Can you work these out from the model? Positions are in its coordinate system, mm. Give positions to 0.01 mm unless a question says otherwise; leave off trailing zeros. Loops run counter-clockwise (first coordinate to the right, second up) from the corner with the lowest first, then second, coordinate; pieces in that order, holes last. Notation, with made-up numbers: (-31, 25) - (10, 25) arc R5 ccw to (10, 31) - close; hole circle Ø3 at (82.5, 36.5). An arc over 180 degrees is marked (long way). Answer as a JSON object with one key per item and string values.
Autodesk Inventor part; units mm, degrees
ref_plane "YZ Plane" through (0, 0, 0) normal (1, 0, 0) x (0, 1, 0)
ref_plane "XZ Plane" through (0, 0, 0) normal (0, 1, 0) x (-1, 0, 0)
ref_plane "XY Plane" through (0, 0, 0) normal (0, 0, 1) x (1, 0, 0)
sketch "Sketch1" plane through (0, 0, 0) normal (0, 1, 0) x (-1, 0, 0)
  line L0 (0, 0) -> (120, 0)
  line L1 (120, 0) -> (120, -40)
  line L2 (120, -40) -> (0, -40)
  line L3 (0, -40) -> (0, 0)
  circle A0 centre (10, -20) radius 3
  circle A1 centre (110, -10) radius 3
  circle A2 centre (110, -30) radius 3
  dimension "d0" = 120
  dimension "d1" = 40
  dimension "d2" = 6
  dimension "d3" = 10
  dimension "d4" = 20
  dimension "d5" = 6
  dimension "d6" = 10
  dimension "d7" = 6
  dimension "d8" = 20
  dimension "d9" = 10
  dimension "d10" = 10
extrude "Extrusion1" add sketch "Sketch1" along normal blind 6
fillet "Fillet1" radius 5 4 edges at (0, 3, 0) (0, 3, -40) (-120, 3, 0) (-120, 3, -40)
properties part number "EboxTslotMount"
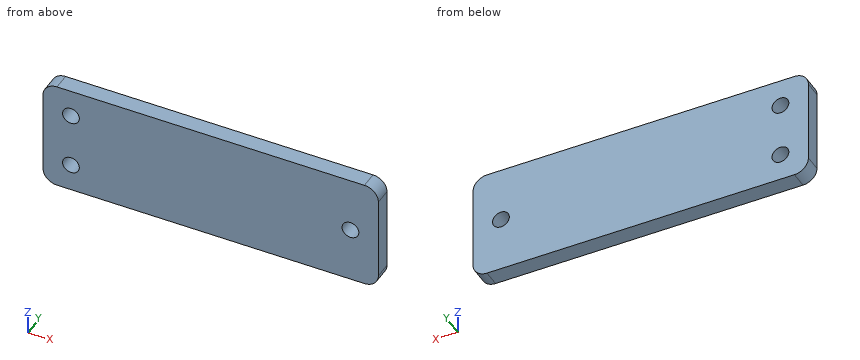
1) I need wall thicknesses on L1, parallel to Z at x = -110, y = 1.75; L2, parallel to Z at x = -10, y = 4.05; L3, parallel to X at y = 3.3, z = -21. Which ranges of each line are inside material? Lowest first, please.
Check sheet entries:
{"L1": "-40 to -33, -27 to -13, -7 to 0", "L2": "-40 to -23, -17 to 0", "L3": "-120 to -12.83, -7.17 to 0"}
2) Imagine slicing it at B-B on x = -10. Write out the boundary of the cut face in (y, z), and give its area (3 significant figures).
Check sheet entries:
{"outline": "(0, -40) - (6, -40) - (6, -23) - (0, -23) - close; (0, -17) - (6, -17) - (6, 0) - (0, 0) - close", "area": "204 mm2"}
3) Imagine slicing it at D-D on x = -110. Write out the boundary of the cut face in (y, z), and give its area (3 significant figures).
Check sheet entries:
{"outline": "(0, -40) - (6, -40) - (6, -33) - (0, -33) - close; (0, -27) - (6, -27) - (6, -13) - (0, -13) - close; (0, -7) - (6, -7) - (6, 0) - (0, 0) - close", "area": "168 mm2"}
4) I'm going to push a flat-ended pin straight in: P1, Ø5.5, axis at x = -110, z = -30, coming from the -Y side. Where does the tip first touch, or does it pass through?
Check sheet entries:
{"P1": "through"}
5) Imagine slicing it at C-C on z = -20. Write out the boundary of the cut face in (x, y).
Check sheet entries:
{"outline": "(-120, 0) - (-13, 0) - (-13, 6) - (-120, 6) - close; (-7, 0) - (0, 0) - (0, 6) - (-7, 6) - close"}
6) Imagine slicing it at A-A on y = 3. Write out the boundary of the cut face in (x, z).
Check sheet entries:
{"outline": "(-120, -35) arc R5 ccw to (-115, -40) - (-5, -40) arc R5 ccw to (0, -35) - (0, -5) arc R5 ccw to (-5, 0) - (-115, 0) arc R5 ccw to (-120, -5) - close; hole circle Ø6 at (-110, -30); hole circle Ø6 at (-110, -10); hole circle Ø6 at (-10, -20)"}
